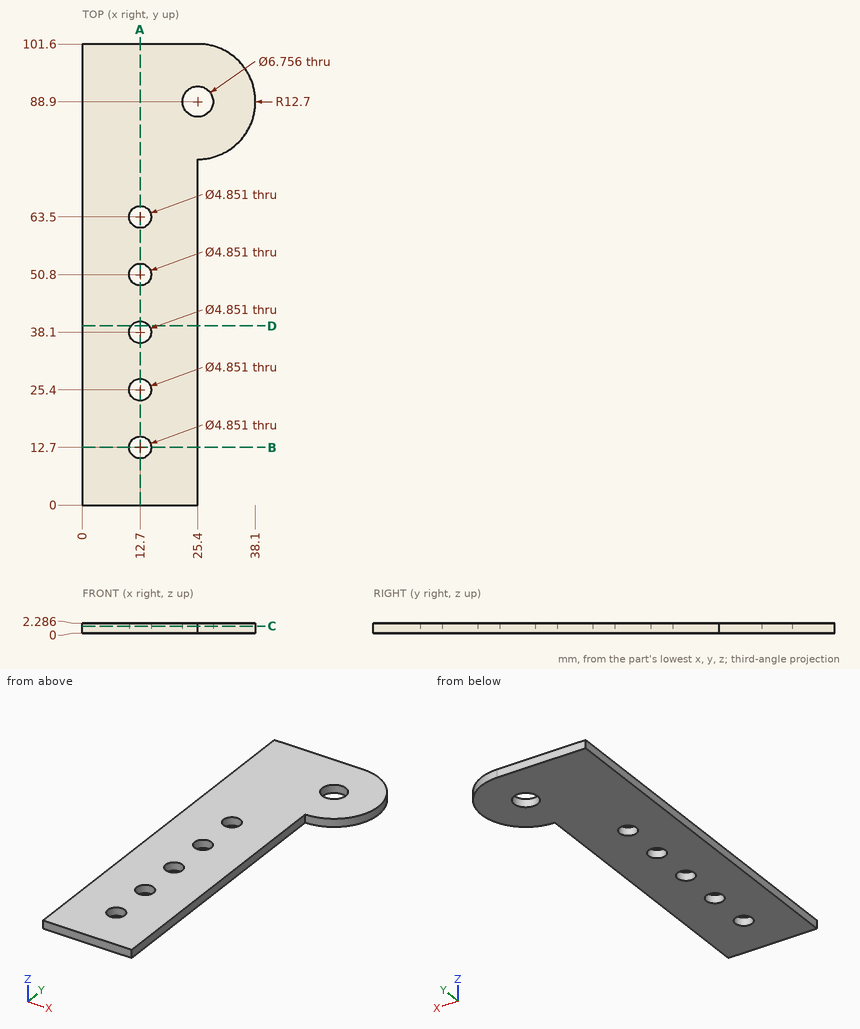
Study the drawing (mm; zero at the part's minimum x, y, z) and answer. Round coordinates to 2 decimals unless told otherwise and drop trailing zeros. Write each loop counter-clockwise with the first axis right and the second up, starting at its lowest first coordinate (ties: lowest second). Pieces come first, ordered by that corner, then holes.
1) A cutting plane is placed at C-C on z = 1.6. Determine the outline of the cut face in (x, y) (1 decimal), and give its area (3 significant figures).
2) Consider probe 1 along Y at (x, z) = (12.7, 1.15) (1 decimal); probe 2 along X at (y, z) = (12.7, 1.2) (1 decimal); probe 3 along Y at (x, z) = (12, 1.65). Determine where each line is inside the solid, lowest interval first.
3) A cutting plane is placed at B-B on y = 12.7. Determine the outline of the cut face in (x, z) (1 decimal).
4) A cutting plane is placed at A-A on x = 12.7. Determine the outline of the cut face in (y, z) (1 decimal).
5) A flat-ended cylindrical pin translates along its axis: P1, Ø1.1, axis at y = 35, z = 1, coming from the +X side. Find the tip coordinate at first contact, or state that the pin passes through.
6) A cutting plane is placed at D-D on y = 39.5. Determine the outline of the cut face in (x, z).
Entries:
1. outline: (0, 0) - (25.4, 0) - (25.4, 76.2) arc R12.7 ccw to (25.4, 101.6) - (0, 101.6) - close; hole circle Ø4.9 at (12.7, 12.7); hole circle Ø4.9 at (12.7, 25.4); hole circle Ø4.9 at (12.7, 38.1); hole circle Ø4.9 at (12.7, 50.8); hole circle Ø4.9 at (12.7, 63.5); hole circle Ø6.8 at (25.4, 88.9)
1. area: 2,710 mm2
2. probe 1: y = 0 to 10.3, 15.1 to 23, 27.8 to 35.7, 40.5 to 48.4, 53.2 to 61.1, 65.9 to 101.6
2. probe 2: x = 0 to 10.3, 15.1 to 25.4
2. probe 3: y = 0 to 10.38, 15.02 to 23.08, 27.72 to 35.78, 40.42 to 48.48, 53.12 to 61.18, 65.82 to 101.6
3. outline: (0, 0) - (10.3, 0) - (10.3, 2.3) - (0, 2.3) - close; (15.1, 0) - (25.4, 0) - (25.4, 2.3) - (15.1, 2.3) - close
4. outline: (0, 0) - (10.3, 0) - (10.3, 2.3) - (0, 2.3) - close; (15.1, 0) - (23, 0) - (23, 2.3) - (15.1, 2.3) - close; (27.8, 0) - (35.7, 0) - (35.7, 2.3) - (27.8, 2.3) - close; (40.5, 0) - (48.4, 0) - (48.4, 2.3) - (40.5, 2.3) - close; (53.2, 0) - (61.1, 0) - (61.1, 2.3) - (53.2, 2.3) - close; (65.9, 0) - (101.6, 0) - (101.6, 2.3) - (65.9, 2.3) - close
5. P1: stops at x = 25.4
6. outline: (0, 0) - (10.72, 0) - (10.72, 2.29) - (0, 2.29) - close; (14.68, 0) - (25.4, 0) - (25.4, 2.29) - (14.68, 2.29) - close
